Design review of the part built by this model. Coordinates are the model's own, in mm. Face numbers are marked on the shaded views. Give positions to 0.01 mm unless a question says otherwise; leave off trailing zeros. Return JSON: item names as keys, results as strings.
```python
from build123d import *

# Parameters (mm, degrees)
F1_DEPTH = 19.05
F0_W     = 12.7
F0_H     = 63.5
F2_DEPTH = 9.525
F0_W_2   = 6.35
F0_H_2   = 31.75
F3_DEPTH = 4.7625
F4_DEPTH = 14.2875


# Not quite as in the source:
# - ends of sketch curves that miss each other by under 0.0002 mm in the source are joined


with BuildPart() as f1:
    # F0 (on Front) → F1 (new body)
    with BuildSketch(Plane.XZ):
        with BuildLine():
            Line((499.03344463, -13.7801575565), (499.03344463, -158.2426575565))
            add(Edge.make_bspline(
                [(499.03344463, -158.2426575565), (534.3674505865, -147.5744416568), (567.5004476082, -131.4772996066), (600.63344463, -115.3801575565)],
                knots=[0.7934300226, 0.7934300226, 0.7934300226, 0.7934300226, 1, 1, 1, 1], degree=3))
            Line((600.63344463, -115.3801575565), (600.63344463, -13.7801575565))
            Line((600.63344463, -13.7801575565), (600.63344463, 87.8198424435))
            add(Edge.make_bspline(
                [(600.63344463, 87.8198424435), (567.5002128258, 103.9114654586), (534.3669810216, 120.0030884738), (499.03344463, 130.6823424435)],
                knots=[0, 0, 0, 0, 0.2065722783, 0.2065722783, 0.2065722783, 0.2065722783], degree=3))
            Line((499.03344463, 130.6823424435), (499.03344463, -13.7801575565))
        make_face()
        with BuildLine():
            Line((169.2494543654, -13.9049269416), (169.2494543653, -198.8486769416))
            add(Edge.make_bspline(
                [(169.2494543653, -198.8486769416), (239.9344955626, -194.7900478461), (311.6955925282, -187.3813112289), (372.03344463, -180.4676575565)],
                knots=[0.2893668435, 0.2893668435, 0.2893668435, 0.2893668435, 0.5700660968, 0.5700660968, 0.5700660968, 0.5700660968], degree=3))
            Line((372.03344463, -180.4676575565), (372.03344463, -13.7801575565))
            Line((372.03344463, -13.7801575565), (372.03344463, 152.9073424435))
            add(Edge.make_bspline(
                [(372.03344463, 152.9073424435), (311.6965969023, 159.7662930053), (239.9327534215, 167.0025918958), (169.2494543654, 171.0388230584)],
                knots=[0.4299386922, 0.4299386922, 0.4299386922, 0.4299386922, 0.7106256488, 0.7106256488, 0.7106256488, 0.7106256488], degree=3))
            Line((169.2494543654, 171.0388230584), (169.2494543654, -13.9049269416))
        make_face()
        with BuildLine():
            Line((372.03344463, -13.7801575565), (372.03344463, -180.4676575565))
            add(Edge.make_bspline(
                [(372.03344463, -180.4676575565), (420.0467519851, -174.9661793441), (460.8268165983, -169.7781895634), (499.03344463, -158.2426575565)],
                knots=[0.5700660968, 0.5700660968, 0.5700660968, 0.5700660968, 0.7934300226, 0.7934300226, 0.7934300226, 0.7934300226], degree=3))
            Line((499.03344463, -158.2426575565), (499.03344463, -13.7801575565))
            Line((499.03344463, -13.7801575565), (499.03344463, 130.6823424435))
            add(Edge.make_bspline(
                [(499.03344463, 130.6823424435), (460.8273243383, 142.2298099053), (420.0485909934, 147.4490938355), (372.03344463, 152.9073424435)],
                knots=[0.2065722783, 0.2065722783, 0.2065722783, 0.2065722783, 0.4299386922, 0.4299386922, 0.4299386922, 0.4299386922], degree=3))
            Line((372.03344463, 152.9073424435), (372.03344463, -13.7801575565))
        make_face()
        with BuildLine():
            Line((-47.06655537, -13.7801514768), (-47.06655537, -204.2801485002))
            add(Edge.make_bspline(
                [(-47.06655537, -204.2801485002), (24.657602579, -203.6563895898), (96.3817605281, -203.0326306794), (169.2494543653, -198.8486769416)],
                knots=[0, 0, 0, 0, 0.2893668435, 0.2893668435, 0.2893668435, 0.2893668435], degree=3))
            Line((169.2494543653, -198.8486769416), (169.2494543654, -13.9049269416))
            Line((169.2494543654, -13.9049269416), (169.2494543654, 171.0388230584))
            add(Edge.make_bspline(
                [(169.2494543654, 171.0388230584), (96.3784736275, 175.1999774928), (24.6559591287, 175.9599115197), (-47.06655537, 176.7198455466)],
                knots=[0.7106256488, 0.7106256488, 0.7106256488, 0.7106256488, 1, 1, 1, 1], degree=3))
            Line((-47.06655537, 176.7198455466), (-47.06655537, -13.7801514768))
        make_face()
    extrude(amount=F1_DEPTH)

    # F0 (on Front) → F2 (join)
    with BuildSketch(Plane.XZ):
        Polygon((-123.26655537, 176.7198455466), (-123.26655537, -13.7801514768), (-104.21655537, -13.7801514768), (-104.21655537, 49.7198424435), (-110.56655537, 49.7198424435), (-110.56655537, 113.2198424435), (-104.21655537, 113.2198424435), (-104.21655537, 176.7198363638), align=None)
        Polygon((-104.21655537, 49.7198424435), (-104.21655537, -13.7801514768), (-85.16655537, -13.7801514768), (-85.16655537, 176.7198455466), (-104.21655537, 176.7198455466), (-104.21655537, 113.2198424435), (-97.86655537, 113.2198424435), (-97.86655537, 49.7198424435), align=None)
        Polygon((-85.16655537, 176.7198455466), (-85.16655537, -13.7801514768), (-72.46655537, -13.7801514768), (-72.46655537, 17.9698485232), (-66.11655537, 17.9698485232), (-66.11655537, 81.4698470349), (-66.11655537, 97.3448462908), (-72.46655537, 97.3448462908), (-72.46655537, 160.8448462908), (-66.11655537, 160.8448462908), (-66.11655537, 176.7198455466), align=None)
        Polygon((-47.06655537, 176.7198455466), (-66.11655537, 176.7198455466), (-66.11655537, 160.8448462908), (-59.76655537, 160.8448462908), (-59.76655537, 97.3448462908), (-66.11655537, 97.3448462908), (-66.11655537, 81.4698470349), (-66.11655537, 17.9698485232), (-59.76655537, 17.9698485232), (-59.76655537, -13.7801514768), (-47.06655537, -13.7801514768), align=None)
        Polygon((-104.21655537, -13.7801514768), (-123.26655537, -13.7801514768), (-123.26655537, -204.2801485003), (-104.21655537, -204.2801485002), (-104.21655537, -140.7801453971), (-110.56655537, -140.7801453971), (-110.56655537, -77.2801453971), (-104.21655537, -77.2801453971), align=None)
        Polygon((-85.16655537, -13.7801514768), (-104.21655537, -13.7801514768), (-104.21655537, -77.2801453971), (-97.86655537, -77.2801453971), (-97.86655537, -140.7801453971), (-104.21655537, -140.7801453971), (-104.21655537, -204.2801393175), (-85.16655537, -204.2801485002), align=None)
        Polygon((-72.46655537, -13.7801514768), (-85.16655537, -13.7801514768), (-85.16655537, -204.2801485002), (-47.06655537, -204.2801485002), (-47.06655537, -13.7801514768), (-59.76655537, -13.7801514768), (-59.76655537, -45.5301514768), (-66.11655537, -45.5301514768), (-72.46655537, -45.5301514768), align=None)
        with Locations((-66.11655537, -156.6551492444)):
            Rectangle(F0_W, F0_H, mode=Mode.SUBTRACT)
    extrude(amount=F2_DEPTH)

    # F0 (on Front) → F3 (join)
    with BuildSketch(Plane.XZ):
        with Locations((-66.11655537, -156.6551492444)):
            Rectangle(F0_W, F0_H)
        with Locations((-69.29155537, -29.6551514768)):
            Rectangle(F0_W_2, F0_H_2)
        with Locations((-62.94155537, -29.6551514768)):
            Rectangle(F0_W_2, F0_H_2)
        with Locations((-69.29155537, 2.0948485232)):
            Rectangle(F0_W_2, F0_H_2)
        with Locations((-62.94155537, 2.0948485232)):
            Rectangle(F0_W_2, F0_H_2)
        Polygon((-66.11655537, 129.0948462908), (-66.11655537, 160.8448462908), (-72.46655537, 160.8448462908), (-72.46655537, 97.3448462908), (-66.11655537, 97.3448462908), align=None)
        Polygon((-59.76655537, 160.8448462908), (-66.11655537, 160.8448462908), (-66.11655537, 129.0948462908), (-66.11655537, 97.3448462908), (-59.76655537, 97.3448462908), align=None)
    extrude(amount=F3_DEPTH)

    # F0 (on Front) → F4 (join)
    with BuildSketch(Plane.XZ):
        Polygon((-104.21655537, 81.4698424435), (-104.21655537, 49.7198424435), (-97.86655537, 49.7198424435), (-97.86655537, 113.2198424435), (-104.21655537, 113.2198424435), align=None)
        Polygon((-110.56655537, 49.7198424435), (-104.21655537, 49.7198424435), (-104.21655537, 81.4698424435), (-104.21655537, 113.2198424435), (-110.56655537, 113.2198424435), align=None)
        with Locations((-107.39155537, -109.0301453971)):
            Rectangle(F0_W_2, F0_H)
        with Locations((-101.04155537, -109.0301453971)):
            Rectangle(F0_W_2, F0_H)
    extrude(amount=F4_DEPTH)


solid = f1.part
```
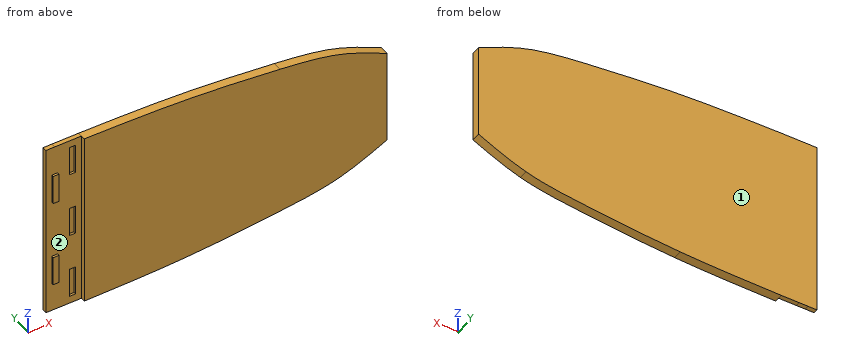
Item 1: For pin 1 (1.4 mm diameter, centred on y = -12.5, z = 93, fed in from -X); pin 2 (1.4 mm diameter, centred on x = -103, y = -12.5, fed in from +Z); pin 3 (1.4 mm diameter, centred on x = -104.5, y = -12.5, fed in from -Z), all flat-tipped, find the tip position at first contact; note any pin that passes through.
Result set:
{"pin 1": "stops at x = -110.57", "pin 2": "stops at z = 113.22", "pin 3": "stops at z = -140.78"}
Item 2: Mouldability with a two-part tool opening along X and no side actions: class the marked faces 1 and 2 as released by +X, released by -X, zero draft, split by the parting line, or undercut.
Result set:
{"face 1": "zero draft", "face 2": "undercut"}
Item 3: Wall thickness on L1, parallel to X at y = -15.5, z = -60.5; L2, parallel to Z at x = 297, y = -4; L3, parallel to Z at x = 536, y = -0.75: over which ranges is each line inside the solid? List them lowest first. Write a range as [from, to].
Result set:
{"L1": "x = [-47.07, 600.63]", "L2": "z = [-188.55, 160.89]", "L3": "z = [-145.04, 117.48]"}
